The listing builds one solid part. Answer for the finished solid, in the listing's coordinates (mm). A direction names the side the tool comes from. Coordinates: 2 decimals unless noted, no trailing zeros. Write each loop counter-clockwise with the first axis right and the second up, starting at its lowest first coordinate (ties: lowest second). Pieces come first, ordered by that corner, then holes. Notation, with made-up numbers: M -26,21 L -16,21 A17 cw -16,30 Z; hole C 63,41 d7. An arc over 180 degrees is marked long. Answer as CSV lines item,"result".
```python
from build123d import *

# Parameters (mm, degrees)
SKETCH1_W           = 2
SKETCH1_H           = 7.3
BOSS_EXTRUDE1_DEPTH = 6
SKETCH3_W           = 16
SKETCH3_H           = 16
BOSS_EXTRUDE3_DEPTH = 2
FILLET2_R           = 0.5


with BuildPart() as part:
    # Sketch1 → Boss-Extrude1 (new body)
    with BuildSketch(Plane(origin=(0, 0, 0), x_dir=(1, 0, 0), z_dir=(0, 1, 0))):
        with Locations((1, 3.65)):
            Rectangle(SKETCH1_W, SKETCH1_H)
    extrude(amount=BOSS_EXTRUDE1_DEPTH)

    # Sketch3 → Boss-Extrude3 (add)
    with BuildSketch(Plane.XY):
        with Locations((1, 3)):
            Rectangle(SKETCH3_W, SKETCH3_H)
    extrude(amount=BOSS_EXTRUDE3_DEPTH)

    # Fillet2
    fillet2_edges = [part.edges().sort_by_distance(p)[0] for p in [
        (-7, 3, 0),
        (-7, 11, 1),
        (1, -5, 0),
        (-7, -5, 1),
        (9, 3, 0),
        (9, -5, 1),
        (1, 11, 0),
        (9, 11, 1),
        (-7, 3, 2),
        (1, -5, 2),
        (9, 3, 2),
        (1, 11, 2),
    ]]
    fillet(fillet2_edges, radius=FILLET2_R)


solid = part.part
```
Q1. Straight lines are drawn through the part: line 1 (Z direction, x = 5.75, y = 9.75); line 2 (Y direction, x = 0.5, z = -5.5). For each, find the intervals that lie inside material, in ascending order.
Output:
line 1,"0 to 2"
line 2,"0 to 6"
Q2. The mould has two halves that part along Z. Classify faces 1 (the flat face through (1, 3, 2)), 2 (the flat face through (1, 6, -4)), 3 (the flat face through (1, 3, -7.3)): pulls with the +Z half, pulls with the -Z half, needs draft (parallel to the pull), parting line crosses it, or undercut.
Output:
face 1,"pulls with the +Z half"
face 2,"needs draft"
face 3,"pulls with the -Z half"
Q3. Find section B-B (x = -0.5). Give the vertices of the cut face in (y, z), and give its area (3 significant figures).
Output:
outline,"M -5,0.5 A0.5 ccw -4.5,0 L 10.5,0 A0.5 ccw 11,0.5 L 11,1.5 A0.5 ccw 10.5,2 L -4.5,2 A0.5 ccw -5,1.5 Z"
area,"31.8 mm2"
Q4. For faces 4 (the flat face through (1, 0, -4)), 5 (the flat face through (0, 3, -4)), 6 (the flat face through (9, 3, 1)), 7 (the flat face through (2, 3, -4)), 8 (the flat face through (1, -5, 1)), determine the directions among +Z, -Z, +X, -X, +Y, -Y from which every point of the face is accessible in a straight line to the end or side of a thin tool.
Output:
face 4,"-Z, +X, -X, -Y"
face 5,"-Z, -X, +Y, -Y"
face 6,"+Z, -Z, +X, +Y, -Y"
face 7,"-Z, +X, +Y, -Y"
face 8,"+Z, -Z, +X, -X, -Y"
Q5. Find section A-A (y = -2.25). Give the vertices of the cut face in (x, z), and give its area (3 significant figures).
Output:
outline,"M -7,0.5 A0.5 ccw -6.5,0 L 8.5,0 A0.5 ccw 9,0.5 L 9,1.5 A0.5 ccw 8.5,2 L -6.5,2 A0.5 ccw -7,1.5 Z"
area,"31.8 mm2"
Q6. Find section D-D (y = 4.5). Give the vertices of the cut face in (x, z).
Output:
outline,"M -7,0.5 A0.5 ccw -6.5,0 L 0,0 L 0,-7.3 L 2,-7.3 L 2,0 L 8.5,0 A0.5 ccw 9,0.5 L 9,1.5 A0.5 ccw 8.5,2 L -6.5,2 A0.5 ccw -7,1.5 Z"
Q7. Find section C-C (z = -6). Give the vertices of the cut face in (x, y), and give its area (3 significant figures).
Output:
outline,"M 0,0 L 2,0 L 2,6 L 0,6 Z"
area,"12.0 mm2"
Q8. Flat-ended cylindrical pins translate along their axes: pin 1 Ø5 at (y, z) = (2.5, -4.5) entering from +X; pin 2 Ø3 at (x, z) = (2, -2) entering from +Y; pin 3 Ø2 at (x, z) = (0.5, -5) entering from -Y. Find the tip coordinate at first contact, or state that the pin passes through.
Output:
pin 1,"x = 2"
pin 2,"y = 6"
pin 3,"y = 0"
